from build123d import *

# Parameters (mm, degrees)
F1_DEPTH = 100


with BuildPart() as f1:
    # F0 (on Top) → F1 (new body)
    with BuildSketch(Plane.XY):
        Polygon((5, 0), (0, 0), (0, -25), (5, -25), (5, -12.5), align=None)
        Polygon((0, 5), (0, 0), (5, 0), (17.5, 0), (50, 0), (50, 5), align=None)
        with BuildLine():
            Line((17.5, 0), (5, 0))
            Line((5, 0), (5, -12.5))
            ThreePointArc((5, -12.5), (8.661165, -3.661165), (17.5, 0))
        make_face()
    extrude(amount=F1_DEPTH)


solid = f1.part
Could you check a few things on this model? Use its own coordinates, in mm. A direction names the side the tool comes from. Coordinates: 2 decimals unless noted, no trailing zeros. Loops run counter-clockwise (first coordinate to the right, second up) from the corner with the lowest first, then second, coordinate; pieces in that order, holes last. Notation, with made-up numbers: (38, 4.5) -> (82, 4.5) arc R20 ccw to (82, 20.5) -> close; hole circle Ø9 at (28.25, 51). An arc over 180 degrees is marked (long way). Answer in a Markdown table with one row per item.
(1) Will these pins go through, and if not, where does the flat tip stop? pin 1 Ø3 at (y, z) = (-14, 23) entering from +X; pin 2 Ø12 at (x, z) = (29, 60) entering from -Y.
Results found:
| item | result |
|---|---|
| pin 1 | stops at x = 5 |
| pin 2 | stops at y = 0 |
(2) If I drill on probe 1 along X at (y, z) = (-19.5, 64); probe 2 along X at (y, z) = (-9.25, 63.5), over which ranges is the centre line in solid material (lowest first)?
Results found:
| item | result |
|---|---|
| probe 1 | x = 0 to 5 |
| probe 2 | x = 0 to 5.43 |
(3) Imagine slicing it at B-B (y = -16.5). List the corners of the cut face in (x, z) for me, plus the area to 3 significant figures.
Results found:
| item | result |
|---|---|
| outline | (0, 0) -> (5, 0) -> (5, 100) -> (0, 100) -> close |
| area | 500 mm^2 |
(4) Imagine slicing it at A-A (z = 61). List the corners of the cut face in (x, y) for me.
Results found:
| item | result |
|---|---|
| outline | (0, -25) -> (5, -25) -> (5, -12.5) arc R12.5 cw to (17.5, 0) -> (50, 0) -> (50, 5) -> (0, 5) -> close |
(5) For faces 1 (the face through (5, -19, 49)), 2 (the face through (50, 2, 49)), which set-ups out of +Z, -Z, +X, -X, +Y, -Y let a thin tool reach every point of the face, with its end or its side?
Results found:
| item | result |
|---|---|
| face 1 | +Z, -Z, +X, -Y |
| face 2 | +Z, -Z, +X, +Y, -Y |
